Geometry check sheet. Reference: the model listing, model coordinates, mm. A direction names the side the tool comes from. Round coordinates to 2 decimals unless told otherwise and drop trailing zeros. Order: outer loops, then holes, each group sorted by start corner. A loop starts at its lowest first (then second) coordinate and runs counter-clockwise, first axis right, second up. Notation, with made-up numbers: (63.5, -27) -> (116.5, -27) arc R24 cw to (116.5, -3) -> close; hole circle Ø1 at (42.25, 89.5). An arc over 180 degrees is marked (long way). Use a Markdown table: item, result. Add a question column.
Item 1: Set-up check for faces 4 (the cylindrical face through (1, -9, 18)), 5 (the cylindrical face through (23.26, -14.33, 7.64)): record each of +Z, -Z, +X, -X, +Y, -Y from which the full face is reachable in a straight line by a thin tool's end or side.
Item 2: Sectioned sample at B-B, the plane y = -14.5. Record the cut outline in (x, z), and give its area (3 significant figures).
Item 3: Gauge pin test, flat ends, axial feed: pin 1 Ø15 at (x, z) = (-15, 5.5) entering from -Y; pin 2 Ø4 at (x, z) = (-15.5, -13.5) entering from -Y; pin 3 Ø10 at (x, y) = (-30, -12) entering from +Z. Record the tip position at first contact, or that the pin passes through.
Item 4: Sectioned sample at A-A, the plane z = 24.5. Record the cut outline in (x, y).
Item 5: Mould release check, pull along X, two halves, no side actions. Record for faces 1 (the cylindrical face through (-2.197, -8.891, -39.498)), 2 (the flat face through (-17, -15.494, 3)), 3 (the flat face through (-1, 0, -3)): pulls with the +X half, pulls with the -X half, needs draft (parallel to the pull), parting line crosses it, or undercut.
Item 6: Sectioned sample at C-C, the plane z = 4. Record the cut outline in (x, y).
Item 7: Material ranges on probe 1 along X at (y, z) = (-17, 9); probe 2 along Y at (x, z) = (9.5, -17); probe 3 along Y at (x, z) = (-26, -25.5), recorded low to high. Write a range as [from, to].
Item 8: Sectioned sample at D-D, the plane y = -5.5. Record the cut outline in (x, z).
from build123d import *

# Parameters (mm, degrees)
F1_DEPTH = 12.7
F4_DEPTH = 2.794
F5_DEPTH = 3.556
F7_DEPTH = 0.508
F8_R     = 4.0932616512
F9_DEPTH = 5.334


with BuildPart() as f1:
    # F0 (on Front) → F1 (new body)
    with BuildSketch(Plane.XZ):
        with BuildLine():
            ThreePointArc((25.0273931209, 30.6353052518), (0.3760595222, 18.0051146813), (-23.726411007, 31.6535899232))
            ThreePointArc((-23.726411007, 31.6535899232), (-0.8260535898, -39.5500944344), (25.0273931209, 30.6353052518))
        make_face()
    extrude(amount=F1_DEPTH)

    # F2 (on face) → F4 (join)
    with BuildSketch(Plane.XZ.offset(12.7)):
        with BuildLine():
            Line((-17.5436979513, 2.6755574061), (-24.6252994984, 0))
            ThreePointArc((-24.6252994984, 0), (-23.4886257248, -2.0111815106), (-21.798320189, -3.5859022896))
            ThreePointArc((-21.798320189, -3.5859022896), (-17.4685188777, -2.3995249593), (-13.1054765957, -3.4571319799))
            ThreePointArc((-13.1054765957, -3.4571319799), (-12.1526852264, 7.9901288569), (-23.6123846381, 7.2009004653))
            Line((-23.6123846381, 7.2009004653), (-17.5436979513, 2.6755574061))
        make_face()
        with BuildLine():
            ThreePointArc((21.5031847078, -3.7765858449), (23.1328376444, 7.7813585574), (11.4750112645, 7.2009004653))
            Line((11.4750112645, 7.2009004653), (17.5436979513, 2.6755574061))
            Line((17.5436979513, 2.6755574061), (10.4620964041, 0))
            ThreePointArc((10.4620964041, 0), (11.5679326814, -1.971798546), (13.2067047826, -3.5291326072))
            ThreePointArc((13.2067047826, -3.5291326072), (17.3835685766, -2.6931747019), (21.5031847078, -3.7765858449))
        make_face()
    extrude(amount=F4_DEPTH)

    # F3 (on face) → F5 (join)
    with BuildSketch(Plane.XZ.offset(12.7)):
        with BuildLine():
            ThreePointArc((-16.6242958605, -13.6971237379), (-18.5050049332, -12.9721756726), (-20.3581005335, -12.1792992577))
            ThreePointArc((-20.3581005335, -12.1792992577), (-22.1561373864, -16.0172531608), (-20.7136999816, -20.0025010854))
            ThreePointArc((-20.7136999816, -20.0025010854), (-18.9311591949, -21.0712313357), (-17.0989353576, -22.052348971))
            Line((-17.0989353576, -22.052348971), (-16.6242958605, -13.6971237379))
        make_face()
        with BuildLine():
            ThreePointArc((-12.6964952724, -14.9659873575), (-14.6722160438, -14.368146145), (-16.6242958605, -13.6971237379))
            Line((-16.6242958605, -13.6971237379), (-17.0989353576, -22.052348971))
            ThreePointArc((-17.0989353576, -22.052348971), (-14.9246231849, -23.0743286561), (-12.6964952724, -23.9729508833))
            Line((-12.6964952724, -23.9729508833), (-12.6964952724, -14.9659873575))
        make_face()
        with BuildLine():
            ThreePointArc((0, -17.0006339589), (-6.4074737383, -16.3528902815), (-12.6964952724, -14.9659873575))
            Line((-12.6964952724, -14.9659873575), (-12.6964952724, -23.9729508833))
            ThreePointArc((-12.6964952724, -23.9729508833), (-10.5399154671, -24.7086802755), (-8.3473040499, -25.3288329734))
            ThreePointArc((-8.3473040499, -25.3288329734), (-4.2048726292, -26.1675803087), (0, -26.5945244967))
            Line((0, -26.5945244967), (0, -17.0006339589))
        make_face()
        with BuildLine():
            ThreePointArc((5.8929180982, -16.9381003904), (2.9472910815, -17.047774638), (0, -17.0006339589))
            Line((0, -17.0006339589), (0, -26.5945244967))
            ThreePointArc((0, -26.5945244967), (2.9481689707, -26.6461592475), (5.8929180982, -26.4950996461))
            Line((5.8929180982, -26.4950996461), (5.8929180982, -16.9381003904))
        make_face()
        with BuildLine():
            ThreePointArc((19.1572063101, -14.4431000637), (12.6013208797, -16.0960178297), (5.8929180982, -16.9381003904))
            Line((5.8929180982, -16.9381003904), (5.8929180982, -26.4950996461))
            ThreePointArc((5.8929180982, -26.4950996461), (9.9769028198, -25.9458134618), (13.9893206769, -25.0071178464))
            ThreePointArc((13.9893206769, -25.0071178464), (16.6026933877, -24.1703555629), (19.1572063101, -23.1681820381))
            Line((19.1572063101, -23.1681820381), (19.1572063101, -14.4431000637))
        make_face()
        with BuildLine():
            ThreePointArc((21.6026995331, -13.6017007753), (20.3848629816, -14.0366713116), (19.1572063101, -14.4431000637))
            Line((19.1572063101, -14.4431000637), (19.1572063101, -23.1681820381))
            ThreePointArc((19.1572063101, -23.1681820381), (20.1276903937, -22.7368350705), (21.0871963633, -22.2815902384))
            ThreePointArc((21.0871963633, -22.2815902384), (23.2235021691, -18.0532138234), (21.6026995331, -13.6017007753))
        make_face()
    extrude(amount=F5_DEPTH)

    # F6 (on face) → F7 (join)
    with BuildSketch(Plane.XZ.offset(12.7)):
        with BuildLine():
            ThreePointArc((0, 7.2009004653), (-11.5972409177, 15.3673055662), (-25.6920997053, 13.7795004994))
            ThreePointArc((-25.6920997053, 13.7795004994), (-32.6858017864, -8.5460763608), (-22.4917009473, -29.6037010849))
            ThreePointArc((-22.4917009473, -29.6037010849), (0.3555994481, -34.9506746467), (23.2028998435, -29.6037010849))
            ThreePointArc((23.2028998435, -29.6037010849), (32.5884250894, -7.1181977593), (23.2028998435, 15.3673055662))
            ThreePointArc((23.2028998435, 15.3673055662), (10.754620627, 13.690167259), (0, 7.2009004653))
        make_face()
    extrude(amount=F7_DEPTH)

    # F8 (on face) → F9 (join)
    with BuildSketch(Plane.XZ.offset(12.7)):
        with BuildLine():
            ThreePointArc((-23.726411007, 31.6535899232), (-0.8260535898, -39.5500944344), (25.0273931209, 30.6353052518))
            ThreePointArc((25.0273931209, 30.6353052518), (0.3760595222, 18.0051146813), (-23.726411007, 31.6535899232))
        make_face()
        with BuildLine():
            ThreePointArc((0, 7.2009004653), (10.754620627, 13.690167259), (23.2028998435, 15.3673055662))
            ThreePointArc((23.2028998435, 15.3673055662), (32.5884250894, -7.1181977593), (23.2028998435, -29.6037010849))
            ThreePointArc((23.2028998435, -29.6037010849), (0.3555994481, -34.9506746467), (-22.4917009473, -29.6037010849))
            ThreePointArc((-22.4917009473, -29.6037010849), (-32.6858017864, -8.5460763608), (-25.6920997053, 13.7795004994))
            ThreePointArc((-25.6920997053, 13.7795004994), (-11.5972409177, 15.3673055662), (0, 7.2009004653))
        make_face(mode=Mode.SUBTRACT)
        with Locations((25.6920978427, 22.4917009473)):
            Circle(F8_R, mode=Mode.SUBTRACT)
    extrude(amount=F9_DEPTH)


solid = f1.part
Found:
| question | item | result |
|---|---|---|
| 1 | face 4 | +Z, +Y, -Y |
| 1 | face 5 | -Y |
| 2 | outline | (-24.63, 0) arc R7.57 ccw to (-21.8, -3.59) arc R8.98 cw to (-13.11, -3.46) arc R7.57 ccw (long way) to (-23.61, 7.2) -> (-17.54, 2.68) -> close; (-23.73, 31.65) arc R39.56 ccw (long way) to (25.03, 30.64) arc R29.19 cw to start; (-20.71, -20) arc R42.89 ccw to (21.09, -22.28) arc R5.96 ccw to (21.6, -13.6) arc R55.4 cw to (-20.36, -12.18) arc R5.54 ccw to start; (10.46, 0) arc R7.57 ccw to (13.21, -3.53) arc R9.45 cw to (21.5, -3.78) arc R7.57 ccw (long way) to (11.48, 7.2) -> (17.54, 2.68) -> close; hole (-25.69, 13.78) arc R31.76 ccw to (-22.49, -29.6) arc R51.49 ccw to (23.2, -29.6) arc R31.63 ccw to (23.2, 15.37) arc R30.93 ccw to (0, 7.2) arc R19.98 ccw to start; hole circle Ø8.19 at (25.69, 22.49) |
| 2 | area | 2,060 mm2 |
| 3 | pin 1 | stops at y = -15.49 |
| 3 | pin 2 | stops at y = -16.26 |
| 3 | pin 3 | stops at z = 30.66 |
| 4 | outline | (-31.06, -18.03) -> (-17.38, -18.03) -> (-17.38, 0) -> (-31.06, 0) -> close; (19.35, -18.03) -> (22.13, -18.03) -> (22.13, -12.7) -> (29.26, -12.7) -> (29.26, -18.03) -> (31.06, -18.03) -> (31.06, 0) -> (19.35, 0) -> close |
| 5 | face 1 | parting line crosses it |
| 5 | face 2 | undercut |
| 5 | face 3 | needs draft |
| 6 | outline | (-39.36, -18.03) -> (-31.09, -18.03) -> (-31.09, -13.21) -> (-19.32, -13.21) -> (-19.32, -15.49) -> (-10.09, -15.49) -> (-10.09, -13.21) -> (15.77, -13.21) -> (15.77, -15.49) -> (25, -15.49) -> (25, -13.21) -> (30.57, -13.21) -> (30.57, -18.03) -> (39.36, -18.03) -> (39.36, 0) -> (-39.36, 0) -> close |
| 7 | probe 1 | x = [-38.52, -28.89], [-1.37, 2.13], [28.17, 38.52] |
| 7 | probe 2 | y = [-16.26, 0] |
| 7 | probe 3 | y = [-13.21, 0] |
| 8 | outline | (-23.73, 31.65) arc R39.56 ccw (long way) to (25.03, 30.64) arc R29.19 cw to start |
